```python
from build123d import *

# Parameters (mm, degrees)
BOSS_EXTRUDE1_DEPTH = 83.125
SKETCH2_W           = 35.157177314
SKETCH2_H           = 3.3
BOSS_EXTRUDE2_DEPTH = 9.8
SKETCH7_W           = 2.5
SKETCH7_H           = 10
BOSS_EXTRUDE4_DEPTH = 83.125
CUT_EXTRUDE5_REACH  = 186.424
SKETCH8_R           = 1.9
CUT_EXTRUDE6_REACH  = 191.835
SKETCH9_R           = 1.9
CUT_EXTRUDE9_REACH  = 182.103
SKETCH12_R          = 1.9
CUT_EXTRUDE7_REACH  = 191.835
SKETCH10_W          = 33.125
SKETCH10_H          = 22
SKETCH10_W_2        = 4.055
SKETCH11_W          = 53.125
SKETCH11_H          = 124.429937858
SKETCH11_H_2        = 13.429202889
CUT_EXTRUDE8_DEPTH  = 5
CHAMFER1_SIZE       = 4
FILLET1_R           = 0.5
CHAMFER2_SIZE       = 10
CHAMFER2_SIZE_2     = 5.773502692


with BuildPart() as part:
    # Sketch1 → Boss-Extrude1 (new body)
    with BuildSketch(Plane(origin=(0, 0, 0), x_dir=(-1, 0, 0), z_dir=(0, 1, 0))):
        Polygon((19.688093764, 147.570616058), (-10.311906236, 2.570616058), (-9.811906236, 2.570616058), (-9.811906236, -4.929383942), (-5.311906236, -4.929383942), (-5.311906236, 2.570616058), (-0.100118033, 2.570616058), (27.83091645, 137.570616058), (69.688093764, 137.570616058), (69.688093764, 147.570616058), align=None)
    extrude(amount=BOSS_EXTRUDE1_DEPTH)

    # Sketch2 → Boss-Extrude2 (add)
    with BuildSketch(Plane(origin=(0, 83.125, 0), x_dir=(-1, 0, 0), z_dir=(0, 1, 0))):
        Polygon((23.871665271, 134.968822427), (-2.701911664, 6.529867237), (-5.933471049, 7.198465731), (20.640105887, 135.63742092), align=None)
        with Locations((48.759505107, 142.570616058)):
            Rectangle(SKETCH2_W, SKETCH2_H)
    boss_extrude2 = extrude(amount=BOSS_EXTRUDE2_DEPTH)

    # Mirror1: Boss-Extrude2 across plane
    add(boss_extrude2.mirror(Plane.ZX.offset(41.5625)))

    # Sketch7 → Boss-Extrude4 (add)
    with BuildSketch(Plane(origin=(0, 83.125, 0), x_dir=(-1, 0, 0), z_dir=(0, 1, 0))):
        Polygon((64.688093764, 137.570616058), (47.188093764, 137.570616058), (47.188093764, 121.570616058), (49.688093764, 121.570616058), (49.688093764, 132.570616058), (62.188093764, 132.570616058), (62.188093764, 115.570616058), (64.688093764, 115.570616058), align=None)
        with Locations((33.438093764, 132.570616058)):
            Rectangle(SKETCH7_W, SKETCH7_H)
    extrude(amount=-BOSS_EXTRUDE4_DEPTH)

    # Sketch8 → Cut-Extrude5 (cut, up to next)
    with BuildSketch(Plane(origin=(-49.688093764, 0, 0), x_dir=(0, -1, 0), z_dir=(-1, 0, 0)), mode=Mode.PRIVATE) as cut_extrude5_sk1:
        with Locations(Location((-72.9725, 124.820616058, 0), (0, 0, 90))):
            Circle(SKETCH8_R)
    cut_extrude5_tool1 = extrude(cut_extrude5_sk1.sketch, amount=-CUT_EXTRUDE5_REACH, mode=Mode.PRIVATE) & part.part
    # Sketch8 → Cut-Extrude5 (cut, up to next)
    with BuildSketch(Plane(origin=(-49.688093764, 0, 0), x_dir=(0, -1, 0), z_dir=(-1, 0, 0)), mode=Mode.PRIVATE) as cut_extrude5_sk2:
        with Locations(Location((-10.1525, 124.820616058, 0), (0, 0, 90))):
            Circle(SKETCH8_R)
    cut_extrude5_tool2 = extrude(cut_extrude5_sk2.sketch, amount=-CUT_EXTRUDE5_REACH, mode=Mode.PRIVATE) & part.part
    add(cut_extrude5_tool1.solids().sort_by_distance((-49.688094, 72.9725, 124.820616))[0], mode=Mode.SUBTRACT)
    add(cut_extrude5_tool2.solids().sort_by_distance((-49.688094, 10.1525, 124.820616))[0], mode=Mode.SUBTRACT)

    # Sketch9 → Cut-Extrude6 (cut, up to next)
    with BuildSketch(Plane(origin=(-64.688093764, 0, 0), x_dir=(0, -1, 0), z_dir=(-1, 0, 0)), mode=Mode.PRIVATE) as cut_extrude6_sk1:
        with Locations(Location((-72.9725, 118.820616058, 0), (0, 0, 90))):
            Circle(SKETCH9_R)
    cut_extrude6_tool1 = extrude(cut_extrude6_sk1.sketch, amount=-CUT_EXTRUDE6_REACH, mode=Mode.PRIVATE) & part.part
    # Sketch9 → Cut-Extrude6 (cut, up to next)
    with BuildSketch(Plane(origin=(-64.688093764, 0, 0), x_dir=(0, -1, 0), z_dir=(-1, 0, 0)), mode=Mode.PRIVATE) as cut_extrude6_sk2:
        with Locations(Location((-18.9025, 118.820616058, 0), (0, 0, 90))):
            Circle(SKETCH9_R)
    cut_extrude6_tool2 = extrude(cut_extrude6_sk2.sketch, amount=-CUT_EXTRUDE6_REACH, mode=Mode.PRIVATE) & part.part
    # Sketch9 → Cut-Extrude6 (cut, up to next)
    with BuildSketch(Plane(origin=(-64.688093764, 0, 0), x_dir=(0, -1, 0), z_dir=(-1, 0, 0)), mode=Mode.PRIVATE) as cut_extrude6_sk3:
        with Locations(Location((-10.1525, 118.820616058, 0), (0, 0, 90))):
            Circle(SKETCH9_R)
    cut_extrude6_tool3 = extrude(cut_extrude6_sk3.sketch, amount=-CUT_EXTRUDE6_REACH, mode=Mode.PRIVATE) & part.part
    # Sketch9 → Cut-Extrude6 (cut, up to next)
    with BuildSketch(Plane(origin=(-64.688093764, 0, 0), x_dir=(0, -1, 0), z_dir=(-1, 0, 0)), mode=Mode.PRIVATE) as cut_extrude6_sk4:
        with Locations(Location((-64.2225, 118.820616058, 0), (0, 0, 90))):
            Circle(SKETCH9_R)
    cut_extrude6_tool4 = extrude(cut_extrude6_sk4.sketch, amount=-CUT_EXTRUDE6_REACH, mode=Mode.PRIVATE) & part.part
    add(cut_extrude6_tool1.solids().sort_by_distance((-64.688094, 72.9725, 118.820616))[0], mode=Mode.SUBTRACT)
    add(cut_extrude6_tool2.solids().sort_by_distance((-64.688094, 18.9025, 118.820616))[0], mode=Mode.SUBTRACT)
    add(cut_extrude6_tool3.solids().sort_by_distance((-64.688094, 10.1525, 118.820616))[0], mode=Mode.SUBTRACT)
    add(cut_extrude6_tool4.solids().sort_by_distance((-64.688094, 64.2225, 118.820616))[0], mode=Mode.SUBTRACT)

    # Sketch12 → Cut-Extrude9 (cut, up to next)
    with BuildSketch(Plane(origin=(-34.688093764, 0, 0), x_dir=(0, -1, 0), z_dir=(-1, 0, 0)), mode=Mode.PRIVATE) as cut_extrude9_sk1:
        with Locations(Location((-72.9725, 130.751875225, 0), (0, 0, 90))):
            Circle(SKETCH12_R)
    cut_extrude9_tool1 = extrude(cut_extrude9_sk1.sketch, amount=-CUT_EXTRUDE9_REACH, mode=Mode.PRIVATE) & part.part
    # Sketch12 → Cut-Extrude9 (cut, up to next)
    with BuildSketch(Plane(origin=(-34.688093764, 0, 0), x_dir=(0, -1, 0), z_dir=(-1, 0, 0)), mode=Mode.PRIVATE) as cut_extrude9_sk2:
        with Locations(Location((-10.1525, 130.751875225, 0), (0, 0, 90))):
            Circle(SKETCH12_R)
    cut_extrude9_tool2 = extrude(cut_extrude9_sk2.sketch, amount=-CUT_EXTRUDE9_REACH, mode=Mode.PRIVATE) & part.part
    add(cut_extrude9_tool1.solids().sort_by_distance((-34.688094, 72.9725, 130.751875))[0], mode=Mode.SUBTRACT)
    add(cut_extrude9_tool2.solids().sort_by_distance((-34.688094, 10.1525, 130.751875))[0], mode=Mode.SUBTRACT)

    # Cut-Extrude7: up to this face of the body (flat: up to its plane)
    cut_extrude7_end = Plane(part.part.faces().sort_by_distance((-32.188093764, 41.5625, 132.621636181))[0])
    # Sketch10 → Cut-Extrude7 (cut, up to the picked face)
    with BuildSketch(Plane(origin=(-64.688093764, 0, 0), x_dir=(0, -1, 0), z_dir=(-1, 0, 0)), mode=Mode.PRIVATE) as cut_extrude7_sk1:
        with Locations((-41.5625, 126.570616058)):
            Rectangle(SKETCH10_W, SKETCH10_H)
    cut_extrude7_tool1 = split(extrude(cut_extrude7_sk1.sketch, amount=-CUT_EXTRUDE7_REACH, mode=Mode.PRIVATE), bisect_by=cut_extrude7_end, keep=Keep.BOTH, mode=Mode.PRIVATE)
    # Sketch10 → Cut-Extrude7 (cut, up to the picked face)
    with BuildSketch(Plane(origin=(-64.688093764, 0, 0), x_dir=(0, -1, 0), z_dir=(-1, 0, 0)), mode=Mode.PRIVATE) as cut_extrude7_sk2:
        with Locations((-81.0975, 126.570616058)):
            Rectangle(SKETCH10_W_2, SKETCH10_H)
    cut_extrude7_tool2 = split(extrude(cut_extrude7_sk2.sketch, amount=-CUT_EXTRUDE7_REACH, mode=Mode.PRIVATE), bisect_by=cut_extrude7_end, keep=Keep.BOTH, mode=Mode.PRIVATE)
    # Sketch10 → Cut-Extrude7 (cut, up to the picked face)
    with BuildSketch(Plane(origin=(-64.688093764, 0, 0), x_dir=(0, -1, 0), z_dir=(-1, 0, 0)), mode=Mode.PRIVATE) as cut_extrude7_sk3:
        with Locations((-2.0275, 126.570616058)):
            Rectangle(SKETCH10_W_2, SKETCH10_H)
    cut_extrude7_tool3 = split(extrude(cut_extrude7_sk3.sketch, amount=-CUT_EXTRUDE7_REACH, mode=Mode.PRIVATE), bisect_by=cut_extrude7_end, keep=Keep.BOTH, mode=Mode.PRIVATE)
    add(cut_extrude7_tool1.solids().sort_by(Axis((-64.688094, 41.5625, 126.570616), (1, 0, 0)))[0], mode=Mode.SUBTRACT)
    add(cut_extrude7_tool2.solids().sort_by(Axis((-64.688094, 81.0975, 126.570616), (1, 0, 0)))[0], mode=Mode.SUBTRACT)
    add(cut_extrude7_tool3.solids().sort_by(Axis((-64.688094, 2.0275, 126.570616), (1, 0, 0)))[0], mode=Mode.SUBTRACT)

    # Sketch11 → Cut-Extrude8 (cut)
    with BuildSketch(Plane(origin=(0.60602789, 0, 0.125385081), x_dir=(0, -1, 0), z_dir=(-0.9792604195071029, 0, -0.20260560403595218))):
        with Locations((-41.5625, 78.141189903)):
            Rectangle(SKETCH11_W, SKETCH11_H)
        with Locations((-41.5625, 9.21161953)):
            Rectangle(SKETCH11_W, SKETCH11_H_2)
    extrude(amount=-CUT_EXTRUDE8_DEPTH, mode=Mode.SUBTRACT)

    # Chamfer1
    chamfer1_edges = [part.edges().sort_by_distance(p)[0] for p in [
        (5.311906236, 41.5625, -4.929383942),
    ]]
    chamfer(chamfer1_edges, length=CHAMFER1_SIZE)

    # Fillet1
    # the kernel refuses this fillet: 0.5 mm, written as the material it takes off along each edge
    with BuildSketch(Plane(origin=(10.311906236, -1.502988145, 2.570616058), x_dir=(-1, 0, 0), z_dir=(0, 1, 0))) as fillet1_piece_1:
        with BuildLine():
            CenterArc((0.611435738, 0.487423918), FILLET1_R, 168.310630825, 88.811624366)
            Line((0.121805528, 0.58872672), (0.112012924, 0.590752776))
            Line((0.112012924, 0.590752776), (-0.009792604, 0.002026056))
            Line((-0.009792604, 0.002026056), (0, -0.01))
            ThreePointArc((0, -0.01), (0.25, -0.01), (0.497771285, -0.009748478))
            Line((0.497771285, -0.009748478), (0.5, 0))
        make_face()
    extrude(amount=86.13097629, mode=Mode.SUBTRACT)

    # Chamfer2
    # the kernel refuses this chamfer: 10, 5.773502692 mm, written as the material it takes off along each edge
    with BuildSketch(Plane(origin=(0.100118033, 68.125, 2.570616058), x_dir=(-0.018925936601608705, 0.9998132206222079, -0.003915711021022488), z_dir=(-0.20260560403595218, 0, 0.9792604195071029))) as chamfer2_piece_1_section:
        Polygon((CHAMFER2_SIZE * 0.999813220622, -CHAMFER2_SIZE * 0.0193267656127), (-CHAMFER2_SIZE_2 * 0.0193267656124, -CHAMFER2_SIZE_2 * 0.999813220604), (0, 0), align=None)
    chamfer2_piece_1 = extrude(amount=137.859140746, mode=Mode.PRIVATE)
    chamfer2_piece_1 = split(chamfer2_piece_1, bisect_by=Plane(origin=(4.844173208, 72.725966315, 4.319504201), z_dir=(-0.9792604195071029, 0, -0.20260560403595218)), keep=Keep.TOP, mode=Mode.PRIVATE)
    add(chamfer2_piece_1, mode=Mode.SUBTRACT)
    with BuildSketch(Plane(origin=(0.100118033, 15, 2.570616058), x_dir=(-0.01892593660160869, -0.9998132206222079, -0.0039157110210224855), z_dir=(-0.20260560403595218, 0, 0.9792604195071029))) as chamfer2_piece_2_section:
        Polygon((CHAMFER2_SIZE * 0.999813220622, CHAMFER2_SIZE * 0.0193267656127), (-CHAMFER2_SIZE_2 * 0.0193267656124, CHAMFER2_SIZE_2 * 0.999813220604), (0, 0), align=None)
    chamfer2_piece_2 = extrude(amount=137.859140746, mode=Mode.PRIVATE)
    chamfer2_piece_2 = split(chamfer2_piece_2, bisect_by=Plane(origin=(4.844173208, 10.399033685, 4.319504201), z_dir=(-0.9792604195071029, 0, -0.20260560403595218)), keep=Keep.TOP, mode=Mode.PRIVATE)
    add(chamfer2_piece_2, mode=Mode.SUBTRACT)


solid = part.part
```
Read the model definition and answer for the solid it produces. Units are mm, in the model's axes. A direction names the side the tool comes from. Coordinates: 2 decimals unless noted, no trailing zeros. Order: outer loops, then holes, each group sorted by start corner. A loop starts at its lowest first (then second) coordinate and runs counter-clockwise, first axis right, second up. Notation, with made-up numbers: (30.25, 35) - (85.25, 35) arc R27 ccw to (85.25, 71) - close; hole circle Ø11 at (-24.5, -16.75). An arc over 180 degrees is marked (long way). Answer as a JSON object with one key per item and string values. Group by question number.
Item 1: Section B-B (y = 47) is taken. Give the vertices of the cut face in (x, z).
Item 2: Section D-D (x = -60.5) is taken. Give the vertices of the cut face in (y, z) (3 decimals).
Item 3: Flat-ended cylindrical pins translate along their axes: P1, Ø5, axis at y = 10.15, z = 118.82, coming from the -X side; P2, Ø14, axis at x = -53.5, z = 130, coming from the +Y side; P3, Ø8, axis at x = -48.5, y = -4.5, coming from the +Z side; P4, Ø4, axis at x = -22, z = 97, coming from the -Y side. Find the tip coordinate at first contact, or state that the pin passes through.
Item 4: Section A-A (x = -40.5) is taken. Give the vertices of the cut face in (y, z) (3 decimals), plus the area to 3 significant figures.
Item 5: A tool of negligible diameter and unlimited length cuts with its end or side. For faces 1 (the face through (-49, 88, 140.921)), 2 (the face through (-66.338, -5, 143)), 3 (the face through (3, 41, 2.571)), 4 (the face through (-49.688, 15, 127)), from which of +Z, -Z, +X, -X, +Y, -Y can it reach the whole face along a straight path? Write none if from no direction.
Item 6: Consider probe 1 along Z at (x, y) = (-44.5, 46.5); probe 2 along Y at (x, z) = (3, 23.5) (3 decimals); probe 3 along Y at (x, z) = (0, 10) (3 decimals). Determine where each line is inside the solid, lowest interval first. Write a range as from..to.
Item 7: Section C-C (z = 54) is taken. Give the vertices of the cut face in (x, y) (1 decimal).
Item 8: The mould has two halves that part along X. Classify faces 5 (the face through (4.3, -4.83, 6.86)), 6 (the face through (-48, 41, 137.571)), 7 (the face through (-18, 83.125, 94)): +X half, -X half, draft (parallel to the pull), parting line (faces both ways), or undercut.
Results are:
{
 "1": {"outline": "(-69.69, 137.57) - (-27.83, 137.57) - (-22.93, 138.58) - (5, 3.58) - (0.1, 2.57) - (5.31, 2.57) - (5.31, -0.93) - (9.31, -4.93) - (9.81, -4.93) - (9.81, 2.57) arc R0.5 ccw to (10.19, 3.16) - (-19.69, 147.57) - (-69.69, 147.57) - close"},
 "2": {"outline": "(-9.8, 140.921) - (0, 140.921) - (0, 137.571) - (4.055, 137.571) - (4.055, 132.571) - (25, 132.571) - (25, 137.571) - (58.125, 137.571) - (58.125, 132.571) - (79.07, 132.571) - (79.07, 137.571) - (83.125, 137.571) - (83.125, 140.921) - (92.925, 140.921) - (92.925, 144.221) - (83.125, 144.221) - (83.125, 147.571) - (0, 147.571) - (0, 144.221) - (-9.8, 144.221) - close"},
 "3": {"P1": "stops at x = -64.69", "P2": "stops at y = 79.07", "P3": "stops at z = 144.22", "P4": "passes through"},
 "4": {"outline": "(-9.8, 140.921) - (0, 140.921) - (0, 137.571) - (83.125, 137.571) - (83.125, 140.921) - (92.925, 140.921) - (92.925, 144.221) - (83.125, 144.221) - (83.125, 147.571) - (0, 147.571) - (0, 144.221) - (-9.8, 144.221) - close", "area": "896 mm^2"},
 "5": {"face 1": "-Z, +X, -X, +Y", "face 2": "+Z, -Z, -X, -Y", "face 3": "-Z, -X, +Y, -Y", "face 4": "-Z, +Y, -Y"},
 "6": {"probe 1": "z = 137.57..147.57", "probe 2": "y = 0..83.125", "probe 3": "y = 0..7.437, 75.688..83.125"},
 "7": {"outline": "(-10.5, 0) - (-7.1, 0) - (-7.1, -9.8) - (-3.7, -9.8) - (-3.7, 0) - (-0.3, 0) - (-0.3, 83.1) - (-3.7, 83.1) - (-3.7, 92.9) - (-7.1, 92.9) - (-7.1, 83.1) - (-10.5, 83.1) - (-10.5, 78.1) - (-5.4, 69.5) - (-5.4, 13.7) - (-10.5, 5) - close"},
 "8": {"face 5": "+X half", "face 6": "undercut", "face 7": "draft"}
}
